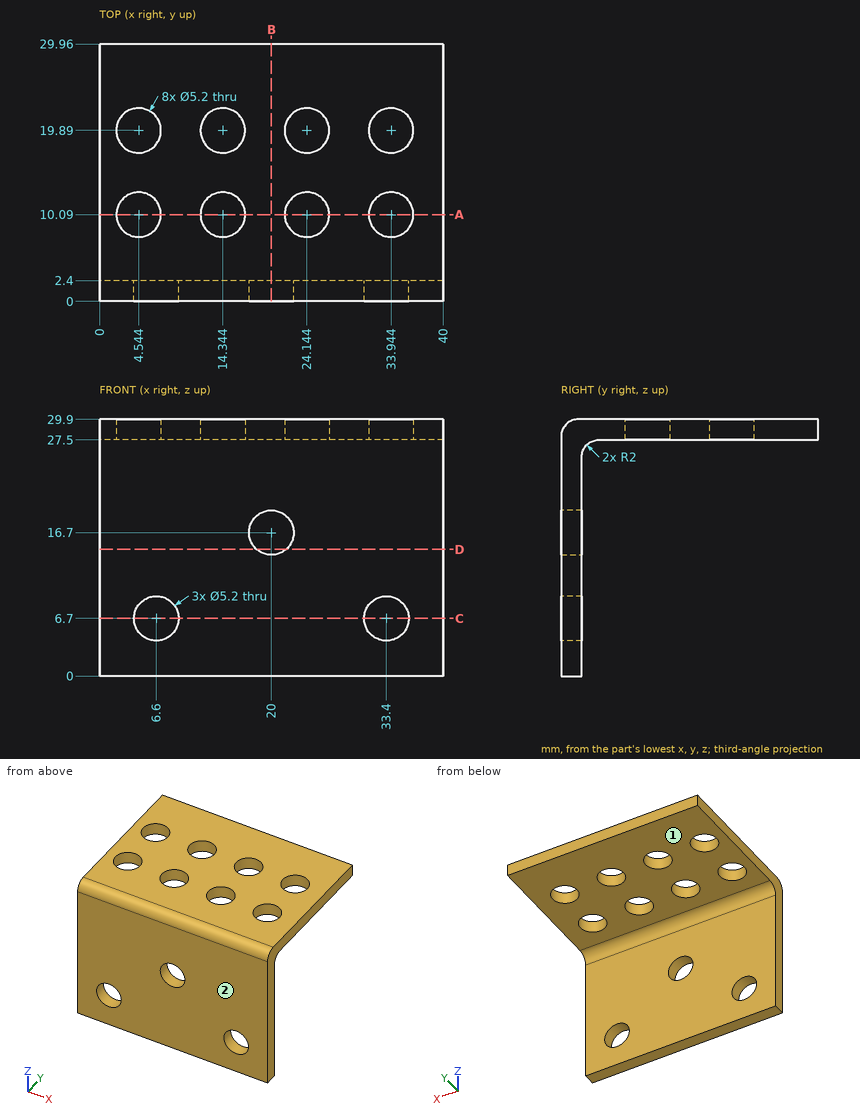
Check sheet for the drawn part. Datum: minimum x, y, z corner. Units: mm. A direction names the side the tool comes from. Give positions to 0.01 mm unless a question says otherwise; leave off trailing zeros. Order: outer loops, then holes, each group sorted by start corner. A loop starts at its lowest first (then second) coordinate and runs counter-clockwise, first axis right, second up. Notation, with made-up numbers: (82.25, 28.5) - (100.25, 28.5) arc R10 ccw to (100.25, 32.5) - close; hole circle Ø5 at (17.25, 35). An arc over 180 degrees is marked (long way). Write item = value, one per line. Start each with the question number.
1) Scan lines: L1, parallel to X at y = 1.5, z = 6.7; L2, parallel to X at y = 10.09, z = 28.45; L3, parallel to Z at x = 9.5, y = 14. Record each from-to range of solid material in increasing order.
2) Section check C-C (z = 6.7). Enter the section's corners in (x, y).
3) Access from +Z, -Z, +X, -X, +Y, -Y to the whole of each face (thin tool, end or side, straight path). Record for the marked faces 1 and 2.
4) Section check D-D (z = 14.75). Enter the section's corners in (x, y).
5) Gauge pin test, flat ends, axial feed: pin 1 Ø4 at (x, y) = (25, 16) entering from -Z; pin 2 Ø4 at (x, z) = (20, 16.7) entering from -Y; pin 3 Ø2 at (x, z) = (16, 7) entering from +Y. Record the tip position at first contact, or that the pin passes through.
6) Section check B-B (x = 20). Enter the section's corners in (y, z), then the cut area to 3 significant figures.
7) Section check A-A (y = 10.09). Enter the section's corners in (x, z).
Geometry check:
q1.L1 = 0 to 4, 9.2 to 30.8, 36 to 40
q1.L2 = 0 to 1.94, 7.14 to 11.74, 16.94 to 21.54, 26.74 to 31.34, 36.54 to 40
q1.L3 = 27.5 to 29.9
q2.outline = (0, 0) - (4, 0) - (4, 2.4) - (0, 2.4) - close; (9.2, 0) - (30.8, 0) - (30.8, 2.4) - (9.2, 2.4) - close; (36, 0) - (40, 0) - (40, 2.4) - (36, 2.4) - close
q3.face_1 = -Z, +X, -X, +Y
q3.face_2 = +Z, -Z, +X, -X, -Y
q4.outline = (0, 0) - (18.28, 0) - (18.28, 2.4) - (0, 2.4) - close; (21.72, 0) - (40, 0) - (40, 2.4) - (21.72, 2.4) - close
q5.pin_1 = 27.5
q5.pin_2 = through
q5.pin_3 = 2.4
q6.outline = (0, 0) - (2.4, 0) - (2.4, 14.1) - (0, 14.1) - close; (0, 19.3) - (2.4, 19.3) - (2.4, 25.5) arc R2 cw to (4.4, 27.5) - (29.96, 27.5) - (29.96, 29.9) - (2, 29.9) arc R2 ccw to (0, 27.9) - close
q6.area = 125 mm2
q7.outline = (0, 27.5) - (1.94, 27.5) - (1.94, 29.9) - (0, 29.9) - close; (7.14, 27.5) - (11.74, 27.5) - (11.74, 29.9) - (7.14, 29.9) - close; (16.94, 27.5) - (21.54, 27.5) - (21.54, 29.9) - (16.94, 29.9) - close; (26.74, 27.5) - (31.34, 27.5) - (31.34, 29.9) - (26.74, 29.9) - close; (36.54, 27.5) - (40, 27.5) - (40, 29.9) - (36.54, 29.9) - close
